Geometry: final body of the model. Coordinates: model frame, mm. A direction names the side the tool comes from. Round coordinates to 2 decimals unless told otherwise and drop trailing zeros. Write each loop counter-clockwise with the first axis right and the second up, starting at its lowest first coordinate (ties: lowest second). Pieces come first, ordered by that corner, then holes. Notation, with made-up numbers: M 54.5,-5 L 110.5,-5 A18 cw 110.5,23 Z; hole C -2,46.25 d4. An arc over 180 degrees is marked long. Use one line per item in the form item = value. Start each with the question number.
Item 1: Pin query (flat end, axial travel): pin 1 Ø0.8 at (y, z) = (1.5, -2) entering from +X; pin 2 Ø3.5 at (x, z) = (18, 0.5) entering from +Y; pin 3 Ø5.5 at (x, z) = (-0.5, -0.5) entering from +Y; pin 4 Ø9 at (x, z) = (46.5, 1.5) entering from +Y. Return the tip coordinate at first contact, or that it passes through.
Item 2: Pull-direction query (X, two-part tool) for faces 4 (the flat face through (1, 5, -5)), 5 (the flat face through (-1, 0, 0)), 6 (the flat face through (-52.75, 3, 0)); classes: pulls with the +X half, pulls with the -X half, needs draft (parallel to the pull), parting line crosses it, or undercut.
Item 3: Reachability of faces 1 (the flat face through (-1, 5, 5)), 2 (the flat face through (49, 2, 0)), 3 (the flat face through (-40.75, 4, 0)) from +Z, -Z, +X, -X, +Y, -Y: full face, straight path, thin tool, end or side. Return the list, or none.
Item 4: Section query B-B (x = 12). Return loops of the section in (y, z).
Item 5: Section query C-C (z = 0). State how many separate pieces and enclosed holes the cut face has, and give its area (3 significant figures).
Item 6: Ray query, probe 1 along Z at (x, y) = (-12, 5); probe 2 along X at (y, z) = (2.35, 0); probe 3 along Y at (x, z) = (25, 1.5). Return the intervals inside material, ascending.
Item 7: Section query A-A (z = -6). Return loops of the section in (x, y).
from build123d import *

# Parameters (mm, degrees)
SKETCH_1_W          = 105.5
SKETCH_1_H          = 16
EXTRUDE_1_DEPTH     = 5
SKETCH_2_W          = 81.5
SKETCH_2_H          = 2
CUT_EXTRUDE_1_DEPTH = 16
SKETCH_5_R          = 1.5
CUT_EXTRUDE_2_DEPTH = 5
SKETCH_6_R          = 3.3
EXTRUDE_3_DEPTH     = 7
SKETCH_7_R          = 5
SKETCH_7_R_2        = 3.3
EXTRUDE_4_DEPTH     = 5
SKETCH_8_W          = 9
SKETCH_8_H          = 2
CUT_EXTRUDE_3_DEPTH = 16
FILLET_1_R          = 1
FILLET_2_R          = 1


with BuildPart() as part:
    # 草图1 → 凸台-拉伸1 (new body)
    with BuildSketch(Plane(origin=(0, 0, 0), x_dir=(1, 0, 0), z_dir=(0, 1, 0))):
        Rectangle(SKETCH_1_W, SKETCH_1_H)
    extrude(amount=EXTRUDE_1_DEPTH)

    # 草图2 → 切除-拉伸1 (cut)
    with BuildSketch(Plane.XY.offset(8)):
        with Locations((0, 4)):
            Rectangle(SKETCH_2_W, SKETCH_2_H)
    extrude(amount=-CUT_EXTRUDE_1_DEPTH, mode=Mode.SUBTRACT)

    # 草图5 → 切除-拉伸2 (cut)
    with BuildSketch(Plane.XZ):
        with Locations(Location((-47.15, 0, 0), (0, 0, 270))):
            Circle(SKETCH_5_R)
        with Locations(Location((47.15, 0, 0), (0, 0, 270))):
            Circle(SKETCH_5_R)
        with Locations(Location((-19.75, 0, 0), (0, 0, 270))):
            Circle(SKETCH_5_R)
        with Locations(Location((19.75, 0, 0), (0, 0, 270))):
            Circle(SKETCH_5_R)
    extrude(amount=-CUT_EXTRUDE_2_DEPTH, mode=Mode.SUBTRACT)

    # 草图6 → 凸台-拉伸3 (add)
    with BuildSketch(Plane.XZ):
        with BuildLine():
            Line((-47.15, 5), (47.15, 5))
            ThreePointArc((47.15, 5), (52.15, 0), (47.15, -5))
            Line((47.15, -5), (-47.15, -5))
            ThreePointArc((-47.15, -5), (-52.15, 0), (-47.15, 5))
        make_face()
        with Locations(Location((-47.15, 0, 0), (0, 0, 270))):
            Circle(SKETCH_6_R, mode=Mode.SUBTRACT)
        with Locations(Location((47.15, 0, 0), (0, 0, 270))):
            Circle(SKETCH_6_R, mode=Mode.SUBTRACT)
        with BuildLine():
            ThreePointArc((42.846436226, 2.545454545), (42.850402728, 3.047716847), (42.416079849, 3.3))
            Line((42.416079849, 3.3), (-42.416079849, 3.3))
            ThreePointArc((-42.416079849, 3.3), (-42.850402728, 3.047716847), (-42.846436226, 2.545454545))
            ThreePointArc((-42.846436226, 2.545454545), (-42.15, 0), (-42.846436226, -2.545454545))
            ThreePointArc((-42.846436226, -2.545454545), (-42.850402728, -3.047716847), (-42.416079849, -3.3))
            Line((-42.416079849, -3.3), (42.416079849, -3.3))
            ThreePointArc((42.416079849, -3.3), (42.850402728, -3.047716847), (42.846436226, -2.545454545))
            ThreePointArc((42.846436226, -2.545454545), (42.15, 0), (42.846436226, 2.545454545))
        make_face(mode=Mode.SUBTRACT)
    extrude(amount=-EXTRUDE_3_DEPTH)

    # 草图7 → 凸台-拉伸4 (add)
    # profile 1 of 2: a face of its own
    with BuildSketch(Plane.XZ):
        with Locations((-19.75, 0)):
            Circle(SKETCH_7_R)
        with Locations(Location((-19.75, 0, 0), (0, 0, 270))):
            Circle(SKETCH_7_R_2, mode=Mode.SUBTRACT)
    # profile 2 of 2: a face of its own
    with BuildSketch(Plane.XZ):
        with Locations((19.75, 0)):
            Circle(SKETCH_7_R)
        with Locations(Location((19.75, 0, 0), (0, 0, 270))):
            Circle(SKETCH_7_R_2, mode=Mode.SUBTRACT)
    extrude(amount=-EXTRUDE_4_DEPTH)

    # 草图8 → 切除-拉伸3 (cut)
    with BuildSketch(Plane.XY.offset(8)):
        with Locations((-48.25, 1)):
            Rectangle(SKETCH_8_W, SKETCH_8_H)
        with Locations((48.25, 1)):
            Rectangle(SKETCH_8_W, SKETCH_8_H)
    extrude(amount=-CUT_EXTRUDE_3_DEPTH, mode=Mode.SUBTRACT)

    # 圆角1
    fillet_1_edges = [part.edges().sort_by_distance(p)[0] for p in [
        (-43.75, 0, 0),
        (43.75, 0, 0),
        (52.75, 3.5, 8),
        (-52.75, 3.5, 8),
        (-52.75, 3.5, -8),
        (52.75, 3.5, -8),
    ]]
    fillet(fillet_1_edges, radius=FILLET_1_R)

    # 圆角2
    fillet_2_edges = [part.edges().sort_by_distance(p)[0] for p in [
        (40.75, 5, -6.5),
        (-40.75, 5, -6.5),
        (-40.75, 5, 6.5),
        (40.75, 5, 6.5),
    ]]
    fillet(fillet_2_edges, radius=FILLET_2_R)


solid = part.part
Working result:
q1.pin_1 = 43.75
q1.pin_2 = 5
q1.pin_3 = 3
q1.pin_4 = 7
q2.face_4 = undercut
q2.face_5 = needs draft
q2.face_6 = pulls with the -X half
q3.face_1 = +Z, +Y
q3.face_2 = +Z, -Z, +X, -Y
q3.face_3 = +Y
q4.outline = M 0,-8 L 3,-8 L 3,-5 L 7,-5 L 7,-3.3 L 3,-3.3 L 3,3.3 L 7,3.3 L 7,5 L 3,5 L 3,8 L 0,8 Z
q5.separate_pieces = 5
q5.enclosed_holes = 0
q5.area = 319 mm²
q6.probe_1 = -5 to -3.3, 3.3 to 5
q6.probe_2 = -52.75 to -48.65, -45.65 to -21.25, -18.25 to 18.25, 21.25 to 45.65, 48.65 to 52.75
q6.probe_3 = 0 to 3
q7.outline = M -52.75,2 L -43.75,2 L -43.75,1 A1 ccw -42.75,0 L 42.75,0 A1 ccw 43.75,1 L 43.75,2 L 52.75,2 L 52.75,5 L 41.75,5 A1 ccw 40.75,4 L 40.75,3 L -40.75,3 L -40.75,4 A1 ccw -41.75,5 L -52.75,5 Z
